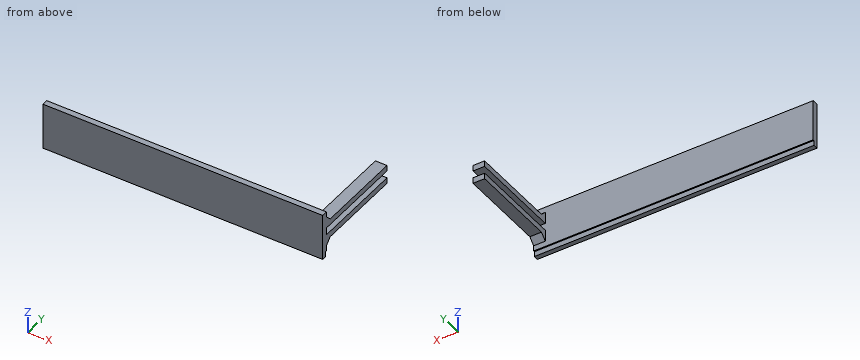
from build123d import *

# Parameters (mm, degrees)
SKETCH1_W           = 152.4
SKETCH1_H           = 25.4
BOSS_EXTRUDE1_DEPTH = 3.175
SKETCH2_W           = 152.4
SKETCH2_H           = 2.794
CUT_EXTRUDE1_DEPTH  = 0.635
SKETCH4_W           = 3.175
SKETCH4_H           = 50.8
BOSS_EXTRUDE2_DEPTH = 6.35
CHAMFER2_SIZE       = 3.175


with BuildPart() as part:
    # Sketch1 → Boss-Extrude1 (new body)
    with BuildSketch(Plane(origin=(0, 0, 0), x_dir=(1, 0, 0), z_dir=(0, 1, 0))):
        with Locations((76.2, 12.7)):
            Rectangle(SKETCH1_W, SKETCH1_H)
    extrude(amount=BOSS_EXTRUDE1_DEPTH)

    # Sketch2 → Cut-Extrude1 (cut)
    with BuildSketch(Plane(origin=(0, 3.175, 0), x_dir=(1, 0, 0), z_dir=(0, 1, 0))):
        with Locations((76.2, 24.003)):
            Rectangle(SKETCH2_W, SKETCH2_H)
    extrude(amount=-CUT_EXTRUDE1_DEPTH, mode=Mode.SUBTRACT)

    # Sketch4 → Boss-Extrude2 (add)
    with BuildSketch(Plane(origin=(152.4, 0, 0), x_dir=(0, 0, -1), z_dir=(1, 0, 0))):
        with Locations((7.747, 28.575)):
            Rectangle(SKETCH4_W, SKETCH4_H)
        with Locations((14.859, 28.575)):
            Rectangle(SKETCH4_W, SKETCH4_H)
    extrude(amount=-BOSS_EXTRUDE2_DEPTH)

    # Chamfer2
    chamfer2_edges = [part.edges().sort_by_distance(p)[0] for p in [
        (149.225, 3.175, -6.1595),
        (149.225, 3.175, -16.4465),
    ]]
    chamfer(chamfer2_edges, length=CHAMFER2_SIZE)


solid = part.part
The listing builds one solid part. Answer for the finished solid, in the listing's coordinates (mm). Coordinates: 2 decimals unless noted, no trailing zeros. Loops run counter-clockwise (first coordinate to the right, second up) from the corner with the lowest first, then second, coordinate; pieces in that order, holes last. Notation, with made-up numbers: (25, -13.75) -> (40, -13.75) arc R24 ccw to (40, 15.25) -> close; hole circle Ø7 at (-35, 84). An arc over 180 degrees is marked (long way). Write item = value, one per line. Start each with the question number.
1) A cutting plane is placed at B-B (x = 132). Give the vertices of the cut face in (y, z) (3 decimals), then the cut area to 3 significant figures.
2) Straight lines are drawn through the part: line 1 (Y direction, x = 115.5, z = -11.5) (3 decimals); line 2 (Y direction, x = 85.5, z = -23.5); line 3 (X direction, y = 7.5, z = -8). For each, find the intervals that lie inside material, in ascending order. Write a range as from..to.
3) A cutting plane is placed at A-A (y = 37.5). Give the vertices of the cut face in (x, z).
4) Given pin 1 Ø10 at (x, z) = (112, -12.5) entering from +Y (3 decimals); pin 2 Ø3 at (x, y) = (149, 29) entering from -Z; pin 3 Ø1.9 at (x, y) = (150.5, 22.5) entering from +Z, each flat-ended and moving along its own axis, determine where each tip first touches the part or whether it passes through.
Responses:
q1.outline = (0, -25.4) -> (2.54, -25.4) -> (2.54, -22.606) -> (3.175, -22.606) -> (3.175, 0) -> (0, 0) -> close
q1.area = 78.9 mm²
q2.line_1 = 0..3.175
q2.line_2 = 0..2.54
q2.line_3 = 146.05..152.4
q3.outline = (146.05, -16.45) -> (152.4, -16.45) -> (152.4, -13.27) -> (146.05, -13.27) -> close; (146.05, -9.33) -> (152.4, -9.33) -> (152.4, -6.16) -> (146.05, -6.16) -> close
q4.pin_1 = 3.175
q4.pin_2 = -16.45
q4.pin_3 = -6.16
